Autodesk Inventor part; units mm, degrees
ref_plane "YZ Plane" through (0, 0, 0) normal (1, 0, 0) x (0, 1, 0)
ref_plane "XZ Plane" through (0, 0, 0) normal (0, 1, 0) x (-1, 0, 0)
ref_plane "XY Plane" through (0, 0, 0) normal (0, 0, 1) x (1, 0, 0)
sketch "Sketch1" plane through (0, 0, 0) normal (0, 0, 1) x (1, 0, 0)
  circle A0 centre (0, 0) radius 2.25
  circle A1 centre (0, 0) radius 4
  dimension "d0" = 4.5
  dimension "d1" = 8
extrude "Extrusion1" add sketch "Sketch1" along normal blind 9
sketch "Sketch2" plane through (0, 0, 9) normal (0, 0, 1) x (1, 0, 0)
  circle A0 centre (0, 0) radius 4.0023
extrude "Extrusion2" add sketch "Sketch2" along normal blind 3
sketch "Sketch3" plane through (0, 0, 12) normal (0, 0, 1) x (1, 0, 0)
  line L0 (2.4, 0.9) -> (2.4, -0.9)
  line L1 (-2.4, -0.9) -> (-2.4, 0.9)
  line L2 (-0.9, 2.4) -> (0.9, 2.4)
  line L3 (0.9, -2.4) -> (-0.9, -2.4)
  line L4 (-0.9, 2.4) -> (-0.9, 0.9)
  line L5 (-0.9, -2.4) -> (-0.9, -0.9)
  line L6 (0.9, 2.4) -> (0.9, 0.9)
  line L7 (0.9, -2.4) -> (0.9, -0.9)
  line L8 (2.4, -0.9) -> (0.9, -0.9)
  line L9 (-0.9, -0.9) -> (-2.4, -0.9)
  line L10 (-2.4, 0.9) -> (-0.9, 0.9)
  line L11 (0.9, 0.9) -> (2.4, 0.9)
  point P0 (0, 0)
  dimension "d6" = 4.8
  dimension "d7" = 1.8
  dimension "d8" = 2.4
  dimension "d10" = 1.8
  dimension "d11" = 4.8
  dimension "d12" = 2.4
extrude "Extrusion3" add sketch "Sketch3" along normal blind 9
fillet "Fillet1" radius 0.5 2 edges at (-0.9, 2.4, 16.5) (-2.4, 0.9, 16.5)
fillet "Fillet2" radius 0.5 1 edges at (-2.4, -0.9, 16.5)
fillet "Fillet3" radius 0.5 1 edges at (-0.9, -2.4, 16.5)
fillet "Fillet4" radius 0.5 4 edges at (0.9, 2.4, 16.5) (2.4, 0.9, 16.5) (2.4, -0.9, 16.5) (0.9, -2.4, 16.5)
sketch "Sketch5" plane through (0, 0, 0) normal (0, 0, -1) x (-1, 0, 0)
  line L0 (1.2561, 1.8667) -> (-1.2561, 1.8667)
  arc A0 (1.2561, 1.8667) -> (-1.2561, 1.8667) centre (0, 0) ccw
  point P0 (0, 0)
extrude "Extrusion4" add sketch "Sketch5" against normal blind 10
properties part number "Motor_Axle_Adapter"
Here's how the part is built. I have some questions about the finished solid (model axes, mm). A direction names the side the tool comes from. Give positions to 0.01 mm unless a question says otherwise; leave off trailing zeros. Order: outer loops, then holes, each group sorted by start corner. A loop starts at its lowest first (then second) coordinate and runs counter-clockwise, first axis right, second up. Notation, with made-up numbers: (51, -37) - (67, -37) arc R16 ccw to (67, -8) - close; hole circle Ø2 at (11.25, 68.5). An arc over 180 degrees is marked (long way). Answer as a JSON object with one key per item and string values. Group by question number.
Item 1: For P1, Ø0.6, axis at x = 0, z = 15, coming from the +Y side; P2, Ø3, axis at y = 1, z = 5, coming from the +X side; P3, Ø1.1, axis at y = -1.5, z = 17.5, coming from the -X side; P4, Ø3, axis at x = 1, y = 2, coming from the +Z side, each with a flat end and sliding along its axis, tell me the tip position at first contact or that it passes through.
Item 2: If we section it at C-C on z = 2.5: Please give me the cut outline in (x, y), and give its area (3 significant figures).
Item 3: Which directions (+Z, -Z, +X, -X, +Y, -Y) give clear straight access to the entire face, cutting with the end or side of a thin tool? Please do faces 1 (the flat face through (2, -2, 12)), 2 (the flat face through (-0.9, -1.4, 16.4)), 3 (the flat face through (1.4, -0.9, 16.4)), 4 (the flat face through (0, 0, 9)), 5 (the flat face through (0.9, 1.4, 16.4)).
Item 4: Please list where these lines run through material, in increasing order: probe 1 along Z at (x, y) = (0.25, 3.75); probe 2 along Y at (x, z) = (-2, 2.75); probe 3 along Z at (x, y) = (1.5, 1.5).
Item 5: If we mould it in two halves opening along X, with no side actions, what happens to faces 6 (the flat face through (0.9, -1.4, 16.4)), 7 (the flat face through (0, 0, 21)), 8 (the cylindrical face through (0.08, -2.25, 4.44))? For each: pulls with the +X half, pulls with the -X half, needs draft (parallel to the pull), parting line crosses it, or undercut.
Result set:
{
 "1": {"P1": "y = 2.4", "P2": "x = 4", "P3": "x = -0.9", "P4": "z = 21"},
 "2": {"outline": "circle Ø8 at (0, 0); hole (-1.26, 1.87) arc R2.25 ccw (long way) to (1.26, 1.87) - close", "area": "35.0 mm²"},
 "3": {"face 1": "+Z", "face 2": "+Z, -X, -Y", "face 3": "+Z, +X, -Y", "face 4": "-Z", "face 5": "+Z, +X, +Y"},
 "4": {"probe 1": "0 to 12", "probe 2": "-3.46 to -1.03, 1.03 to 3.46", "probe 3": "9 to 12"},
 "5": {"face 6": "pulls with the +X half", "face 7": "needs draft", "face 8": "undercut"}
}
